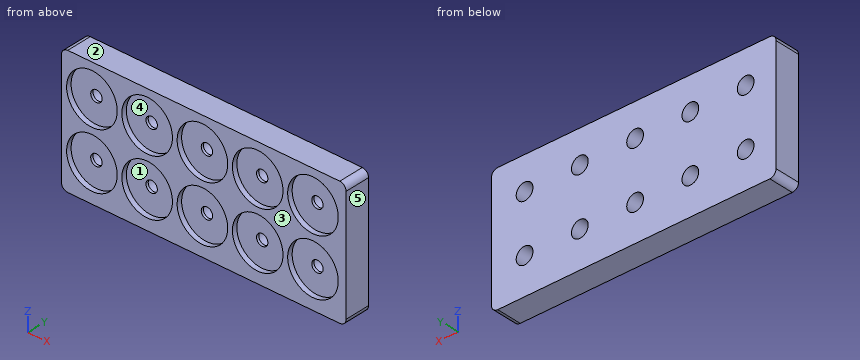
```python
from build123d import *

# Parameters (mm, degrees)
BOSS_EXTRUDE1_DEPTH = 50.8
SKETCH2_R           = 50.8
CUT_EXTRUDE1_DEPTH  = 10.16
SKETCH3_R           = 11.43
CUT_EXTRUDE2_DEPTH  = 627.721516784
SKETCH7_R           = 16.8275
CUT_EXTRUDE3_DEPTH  = 35.56


with BuildPart() as part:
    # Sketch1 → Boss-Extrude1 (new body)
    with BuildSketch(Plane(origin=(0, 0, 0), x_dir=(1, 0, 0), z_dir=(0, 1, 0))):
        with BuildLine():
            Line((-12.7, 0), (-558.8, 0))
            ThreePointArc((-558.8, 0), (-567.780256121, 3.719743879), (-571.5, 12.7))
            Line((-571.5, 12.7), (-571.5, 241.3))
            ThreePointArc((-571.5, 241.3), (-567.780256121, 250.280256121), (-558.8, 254))
            Line((-558.8, 254), (-12.7, 254))
            ThreePointArc((-12.7, 254), (-3.719743879, 250.280256121), (0, 241.3))
            Line((0, 241.3), (0, 12.7))
            ThreePointArc((0, 12.7), (-3.719743879, 3.719743879), (-12.7, 0))
        make_face()
    extrude(amount=BOSS_EXTRUDE1_DEPTH)

    # Sketch2 → Cut-Extrude1 (cut)
    with BuildSketch(Plane(origin=(0, 0, 0), x_dir=(1, 0, 0), z_dir=(0, 1, 0))):
        with Locations(Location((-177.499611663, 66.04, 0), (0, 0, 270))):
            Circle(SKETCH2_R)
        with Locations(Location((-66.57081555, 66.04, 0), (0, 0, 270))):
            Circle(SKETCH2_R)
        with Locations(Location((-288.428407775, 66.04, 0), (0, 0, 270))):
            Circle(SKETCH2_R)
        with Locations(Location((-399.357203888, 66.04, 0), (0, 0, 270))):
            Circle(SKETCH2_R)
        with Locations(Location((-510.286, 66.04, 0), (0, 0, 270))):
            Circle(SKETCH2_R)
        with Locations(Location((-177.499611663, 180.34, 0), (0, 0, 270))):
            Circle(SKETCH2_R)
        with Locations(Location((-288.428407775, 180.34, 0), (0, 0, 270))):
            Circle(SKETCH2_R)
        with Locations(Location((-399.357203888, 180.34, 0), (0, 0, 270))):
            Circle(SKETCH2_R)
        with Locations(Location((-510.286, 180.34, 0), (0, 0, 270))):
            Circle(SKETCH2_R)
        with Locations(Location((-66.57081555, 180.34, 0), (0, 0, 270))):
            Circle(SKETCH2_R)
    extrude(amount=CUT_EXTRUDE1_DEPTH, mode=Mode.SUBTRACT)

    # Sketch3 → Cut-Extrude2 (cut, through all)
    with BuildSketch(Plane.XZ.offset(-10.16)):
        with Locations(Location((-66.57081555, -180.34, 0), (0, 0, 270))):
            Circle(SKETCH3_R)
        with Locations(Location((-177.499611663, -180.34, 0), (0, 0, 270))):
            Circle(SKETCH3_R)
        with Locations(Location((-288.428407775, -180.34, 0), (0, 0, 270))):
            Circle(SKETCH3_R)
        with Locations(Location((-399.357203888, -180.34, 0), (0, 0, 270))):
            Circle(SKETCH3_R)
        with Locations(Location((-510.286, -180.34, 0), (0, 0, 270))):
            Circle(SKETCH3_R)
        with Locations(Location((-510.286, -66.04, 0), (0, 0, 90))):
            Circle(SKETCH3_R)
        with Locations(Location((-399.357203888, -66.04, 0), (0, 0, 90))):
            Circle(SKETCH3_R)
        with Locations(Location((-288.428407775, -66.04, 0), (0, 0, 90))):
            Circle(SKETCH3_R)
        with Locations(Location((-177.499611663, -66.04, 0), (0, 0, 90))):
            Circle(SKETCH3_R)
        with Locations(Location((-66.57081555, -66.04, 0), (0, 0, 90))):
            Circle(SKETCH3_R)
    extrude(amount=-CUT_EXTRUDE2_DEPTH, mode=Mode.SUBTRACT)

    # Sketch7 → Cut-Extrude3 (cut)
    with BuildSketch(Plane(origin=(0, 50.8, 0), x_dir=(1, 0, 0), z_dir=(0, 1, 0))):
        with Locations(Location((-66.57081555, 180.34, 0), (0, 0, 270))):
            Circle(SKETCH7_R)
        with Locations(Location((-66.57081555, 66.04, 0), (0, 0, 270))):
            Circle(SKETCH7_R)
        with Locations(Location((-177.499611663, 66.04, 0), (0, 0, 270))):
            Circle(SKETCH7_R)
        with Locations(Location((-288.428407775, 66.04, 0), (0, 0, 270))):
            Circle(SKETCH7_R)
        with Locations(Location((-399.357203888, 66.04, 0), (0, 0, 270))):
            Circle(SKETCH7_R)
        with Locations(Location((-510.286, 66.04, 0), (0, 0, 270))):
            Circle(SKETCH7_R)
        with Locations(Location((-177.499611663, 180.34, 0), (0, 0, 270))):
            Circle(SKETCH7_R)
        with Locations(Location((-288.428407775, 180.34, 0), (0, 0, 270))):
            Circle(SKETCH7_R)
        with Locations(Location((-399.357203888, 180.34, 0), (0, 0, 270))):
            Circle(SKETCH7_R)
        with Locations(Location((-510.286, 180.34, 0), (0, 0, 270))):
            Circle(SKETCH7_R)
    extrude(amount=-CUT_EXTRUDE3_DEPTH, mode=Mode.SUBTRACT)


solid = part.part
```
Check sheet for the modelled part. Datum: model origin and axes. Units: mm. Face numbers are marked on the shaded views. A direction names the side the tool comes from. Give positions to 0.01 mm unless a question says otherwise; leave off trailing zeros. Use CSV: the item, a comma, the result in double quotes. Start each with the question number.
1) Sectioned sample at A-A, the plane y = 37. Give the number of separate pieces and of enclosed holes in the cut face, plus the area to 3 significant figures.
2) Mould release check, pull along X, two halves, no side actions. Record for the marked faces 3, 4 and 5: released by +X, released by -X, zero draft, split by the parting line, or undercut.
3) Go/stop test with a flat-tipped pin: P1, Ø4, axis at x = -400.5, z = -146, coming from the -Y side. Record where the tip stops, or that it passes through.
4) Material ranges on line 1 (X direction, y = 30.5, z = -66.04); line 2 (X direction, y = 12, z = -180); line 3 (Z direction, x = -518, y = 13), recorded low to high. Write a range as from..to.
5) Set-up check for the marked faces 1 and 2: record each of +Z, -Z, +X, -X, +Y, -Y from which the full face is reachable in a straight line by a thin tool's end or side.
Recorded:
1,separate pieces,"1"
1,enclosed holes,"10"
1,area,"136,000 mm2"
2,face 3,"zero draft"
2,face 4,"undercut"
2,face 5,"released by +X"
3,P1,"y = 10.16"
4,line 1,"-571.5..-527.11, -493.46..-416.18, -382.53..-305.26, -271.6..-194.33, -160.67..-83.4, -49.74..0"
4,line 2,"-571.5..-521.71, -498.86..-410.78, -387.93..-299.85, -277..-188.92, -166.07..-78, -55.15..0"
4,line 3,"-254..-188.77, -171.91..-74.47, -57.61..0"
5,face 1,"-Y"
5,face 2,"+Z, +X, -X, +Y, -Y"
